The listing builds one solid part. Answer for the finished solid, in the listing's coordinates (mm). A direction names the side the tool comes from. Round coordinates to 2 decimals unless told otherwise and drop trailing zeros. Write each loop counter-clockwise with the first axis right and the second up, starting at its lowest first coordinate (ties: lowest second). Pieces come first, ordered by that corner, then holes. Notation, with made-up numbers: (53, -1.75) - (71, -1.75) arc R27 cw to (71, 15.25) - close; hole circle Ø6 at (-10.5, 65). An arc over 180 degrees is marked (long way). Answer as CSV lines item,"result". Start each with the question number.
Item 1: For a pull along Y with two mould halves and no side action, classify faces 3 (the cylindrical face through (27.545, 9.462, 857.23)), 4 (the flat face through (-32, 0, 913)), 5 (the cylindrical face through (-6.288, 28.852, 858.751)) as pulls with the +Y half, pulls with the -Y half, needs draft (parallel to the pull), parting line crosses it, or undercut.
Item 2: Straight lines are drawn through the part: line 1 along X through (y, z) = (-0.5, 809); line 2 along Y through (x, z) = (-2, 853); line 3 along Z through (x, y) = (4.5, -13.5). For each, find the intervals that lie inside material, in ascending order. Write a range as [from, to].
Item 3: A cutting plane is placed at C-C on y = 0. Determine the outline of the cut face in (x, z), and give its area (3 significant figures).
Item 4: Which of the six approach directions +Z, -Z, +X, -X, +Y, -Y give full straight-line access (tool end or side, diameter ignored) to faces 1 (the flat face through (2, -30, 892.3)), 2 (the flat face through (27, 2, 913))?
Item 5: Flat-ended cylindrical pins translate along their axes: pin 1 (8 mm diameter, centred on x = -7.5, y = -17.5, fed in from +Z); pin 2 (6 mm diameter, centred on x = -1.5, z = 887, fed in from +Y); pin 3 (2 mm diameter, centred on y = -24, z = 872, fed in from -X); pin 4 (4 mm diameter, centred on x = -4, z = 856.5, fed in from -Y). Find the tip coordinate at first contact, or state that the pin passes through.
Item 6: A cutting plane is placed at A-A on x = -2.5. Determine the outline of the cut face in (y, z).
Item 7: A cutting plane is placed at B-B on z = 827. Determine the outline of the cut face in (x, y).
```python
from build123d import *

# Parameters (mm, degrees)
CYLINDER007_R     = 31.5
CYLINDER007_DEPTH = 110
CYLINDER008_R     = 29.1
CYLINDER008_DEPTH = 110
POCKET064_DEPTH   = 20.7


with BuildPart() as part:
    # Cylinder007 → Cylinder007 (join)
    with BuildSketch(Plane.XY.offset(-31)):
        Circle(CYLINDER007_R)
    extrude(amount=CYLINDER007_DEPTH)

    # Cylinder008 → Cylinder008 (cut)
    with BuildSketch(Plane.XY.offset(-28)):
        Circle(CYLINDER008_R)
    extrude(amount=CYLINDER008_DEPTH, mode=Mode.SUBTRACT)

    # Sketch123 (on DatumPlane) → Pocket064 (cut)
    with BuildSketch(Plane.XY.offset(79)):
        Polygon((-20.565207, -6.209014), (-18.868151, -4.511957), (9.318102, -32.69821), (7.621046, -34.395267), align=None)
        Polygon((-18.868151, 4.511957), (-20.565207, 6.209014), (7.621046, 34.395267), (9.318102, 32.69821), align=None)
    extrude(amount=-POCKET064_DEPTH, mode=Mode.SUBTRACT)


with BuildPart() as part_1:
    # Body022024 placement: moved
    add(part.part.moved(Location((-2.5, 0, 834))))


solid = part_1.part
```
Geometry says:
1,face 3,"parting line crosses it"
1,face 4,"needs draft"
1,face 5,"undercut"
2,line 1,"x = [-34, -31.6], [26.6, 29]"
2,line 2,"y = [-31.5, -29.1], [29.1, 31.5]"
2,line 3,"z = [803, 806]"
3,outline,"(-34, 803) - (29, 803) - (29, 913) - (26.6, 913) - (26.6, 806) - (-31.6, 806) - (-31.6, 913) - (-34, 913) - close"
3,area,"703 mm^2"
4,face 1,"+Z"
4,face 2,"+Z, +X, -X, +Y, -Y"
5,pin 1,"stops at z = 806"
5,pin 2,"stops at y = 31.5"
5,pin 3,"stops at x = -24.02"
5,pin 4,"stops at y = -31.5"
6,outline,"(-31.5, 803) - (31.5, 803) - (31.5, 913) - (29.1, 913) - (29.1, 806) - (-29.1, 806) - (-29.1, 913) - (-31.5, 913) - close"
7,outline,"circle Ø63 at (-2.5, 0); hole circle Ø58.2 at (-2.5, 0)"
